```python
from build123d import *

# Parameters (mm, degrees)
SKETCH_W        = 230
SKETCH_H        = 140
PAD_DEPTH       = 40
SKETCH001_W     = 222
SKETCH001_H     = 132
POCKET_DEPTH    = 36
SKETCH002_W     = 98
SKETCH002_H     = 40
POCKET001_DEPTH = 5
SKETCH003_W     = 18
SKETCH003_H     = 12
POCKET002_DEPTH = 5
SKETCH004_W     = 15
SKETCH004_H     = 15
POCKET003_DEPTH = 5
SKETCH005_R     = 5
SKETCH005_R_2   = 1.9
PAD001_DEPTH    = 5
CHAMFER_SIZE    = 2


with BuildPart() as part:
    # Sketch → Pad (new body)
    with BuildSketch(Plane.XY):
        with Locations((115, 70)):
            Rectangle(SKETCH_W, SKETCH_H)
    extrude(amount=PAD_DEPTH)

    # Sketch001 (on Face6 of Pad) → Pocket (cut)
    with BuildSketch(Plane.XY.offset(40)):
        with Locations((115, 70)):
            Rectangle(SKETCH001_W, SKETCH001_H)
    extrude(amount=-POCKET_DEPTH, mode=Mode.SUBTRACT)

    # Sketch002 (on Face4 of Pocket) → Pocket001 (cut)
    with BuildSketch(Plane(origin=(0, 0, 0), x_dir=(1, 0, 0), z_dir=(0, 0, -1))):
        with Locations((171, -40)):
            Rectangle(SKETCH002_W, SKETCH002_H)
    extrude(amount=-POCKET001_DEPTH, mode=Mode.SUBTRACT)

    # Sketch003 (on Face2 of Pocket001) → Pocket002 (cut)
    with BuildSketch(Plane(origin=(0, 0, 0), x_dir=(0, -1, 0), z_dir=(-1, 0, 0))):
        with Locations((-114, 15)):
            Rectangle(SKETCH003_W, SKETCH003_H)
    extrude(amount=-POCKET002_DEPTH, mode=Mode.SUBTRACT)

    # Sketch004 (on Face6 of Pocket002) → Pocket003 (cut)
    with BuildSketch(Plane(origin=(0, 140, 0), x_dir=(-1, 0, 0), z_dir=(0, 1, 0))):
        with Locations((-197.5, 20)):
            Rectangle(SKETCH004_W, SKETCH004_H)
    extrude(amount=-POCKET003_DEPTH, mode=Mode.SUBTRACT)

    # Sketch005 (on Face23 of Pocket003) → Pad001 (join)
    with BuildSketch(Plane.XY.offset(4)):
        with Locations((217.5, 12.5)):
            Circle(SKETCH005_R)
        with Locations((217.5, 12.5)):
            Circle(SKETCH005_R_2, mode=Mode.SUBTRACT)
        with Locations((124.5, 12.5)):
            Circle(SKETCH005_R)
        with Locations((124.5, 12.5)):
            Circle(SKETCH005_R_2, mode=Mode.SUBTRACT)
        with Locations((217.5, 67.5)):
            Circle(SKETCH005_R)
        with Locations((217.5, 67.5)):
            Circle(SKETCH005_R_2, mode=Mode.SUBTRACT)
        with Locations((124.5, 67.5)):
            Circle(SKETCH005_R)
        with Locations((124.5, 67.5)):
            Circle(SKETCH005_R_2, mode=Mode.SUBTRACT)
        with Locations((15, 127.5)):
            Circle(SKETCH005_R)
        with Locations((15, 127.5)):
            Circle(SKETCH005_R_2, mode=Mode.SUBTRACT)
        with Locations((65, 127.5)):
            Circle(SKETCH005_R)
        with Locations((65, 127.5)):
            Circle(SKETCH005_R_2, mode=Mode.SUBTRACT)
        with Locations((65, 103.5)):
            Circle(SKETCH005_R)
        with Locations((65, 103.5)):
            Circle(SKETCH005_R_2, mode=Mode.SUBTRACT)
        with Locations((15, 103.5)):
            Circle(SKETCH005_R)
        with Locations((15, 103.5)):
            Circle(SKETCH005_R_2, mode=Mode.SUBTRACT)
        with Locations((15, 63)):
            Circle(SKETCH005_R)
        with Locations((15, 63)):
            Circle(SKETCH005_R_2, mode=Mode.SUBTRACT)
        with Locations((15, 15)):
            Circle(SKETCH005_R)
        with Locations((15, 15)):
            Circle(SKETCH005_R_2, mode=Mode.SUBTRACT)
        with Locations((83, 15)):
            Circle(SKETCH005_R)
        with Locations((83, 15)):
            Circle(SKETCH005_R_2, mode=Mode.SUBTRACT)
        with Locations((83, 63)):
            Circle(SKETCH005_R)
        with Locations((83, 63)):
            Circle(SKETCH005_R_2, mode=Mode.SUBTRACT)
        with Locations((85, 127.5)):
            Circle(SKETCH005_R)
        with Locations((85, 127.5)):
            Circle(SKETCH005_R_2, mode=Mode.SUBTRACT)
        with Locations((85, 101.5)):
            Circle(SKETCH005_R)
        with Locations((85, 101.5)):
            Circle(SKETCH005_R_2, mode=Mode.SUBTRACT)
        with Locations((151, 101.5)):
            Circle(SKETCH005_R)
        with Locations((151, 101.5)):
            Circle(SKETCH005_R_2, mode=Mode.SUBTRACT)
        with Locations((151, 127.5)):
            Circle(SKETCH005_R)
        with Locations((151, 127.5)):
            Circle(SKETCH005_R_2, mode=Mode.SUBTRACT)
    extrude(amount=PAD001_DEPTH)

    # Chamfer
    chamfer_edges = [part.edges().sort_by_distance(p)[0] for p in [
        (0, 140, 20),
        (115, 140, 0),
        (230, 140, 20),
        (230, 70, 0),
        (230, 0, 20),
        (115, 0, 0),
        (0, 0, 20),
        (0, 70, 0),
    ]]
    chamfer(chamfer_edges, length=CHAMFER_SIZE)


solid = part.part
```
Geometry check sheet. Reference: the model listing, model coordinates, mm. Round coordinates to 2 decimals unless told otherwise and drop trailing zeros. Loops run counter-clockwise (first coordinate to the right, second up) from the corner with the lowest first, then second, coordinate; pieces in that order, holes last. Notation, with made-up numbers: (23.5, 62.5) - (53.5, 62.5) arc R6 ccw to (53.5, 72.5) - close; hole circle Ø5 at (38.25, -10.75). An arc over 180 degrees is marked (long way). Write each question's results on one line, items separated by ' | '. Start each with the question number.
Q1. Cross-section at C-C on x = 23.5. Enter the section's corners in (y, z), and give its area (3 significant figures).
Q2. Cross-section at A-A on z = 15. Enter the section's corners in (x, y), and give its area (3 significant figures).
Q3. Thickness scan on line 1 (Y direction, x = 151, z = 6); line 2 (Y direction, x = 124.5, z = 5.75); line 3 (X direction, y = 19, z = 17). Record the ranges inside material, lowest first. Write a range as [from, to].
Q4. Gauge pin test, flat ends, axial feed: P1, Ø1.5, axis at x = 155.5, y = 59.5, coming from the +Z side; P2, Ø3, axis at x = 219, y = 67, coming from the +Z side; P3, Ø12, axis at x = 184, y = 27, coming from the +Z side. Record the tip position at first contact, or that the pin passes through.
Q5. Release check for a two-part mould opening along X. For faces 1 (the flat face through (113, 0, 21)), 2 (the cylindrical face through (87.619, 13.085, 6.465)) record: +X half, -X half, draft (parallel to the pull), parting line (faces both ways), or undercut.
Q6. Cross-section at B-B on y = 36. Enter the section's corners in (x, z), and give its area (3 significant figures).
Answers below:
1) outline: (0, 2) - (2, 0) - (138, 0) - (140, 2) - (140, 40) - (136, 40) - (136, 4) - (4, 4) - (4, 40) - (0, 40) - close | area: 844 mm²
2) outline: (0, 2) - (2, 0) - (228, 0) - (230, 2) - (230, 138) - (228, 140) - (205, 140) - (205, 136) - (226, 136) - (226, 4) - (4, 4) - (4, 105) - (0, 105) - close; (0, 123) - (4, 123) - (4, 136) - (190, 136) - (190, 140) - (2, 140) - (0, 138) - close | area: 2,760 mm²
3) line 1: y = [0, 4], [96.5, 99.6], [103.4, 106.5], [122.5, 125.6], [129.4, 132.5], [136, 140] | line 2: y = [0, 4], [7.5, 10.6], [14.4, 17.5], [62.5, 65.6], [69.4, 72.5], [136, 140] | line 3: x = [0, 4], [226, 230]
4) P1: stops at z = 4 | P2: stops at z = 9 | P3: passes through
5) face 1: draft | face 2: undercut
6) outline: (0, 2) - (2, 0) - (122, 0) - (122, 4) - (4, 4) - (4, 40) - (0, 40) - close; (220, 0) - (228, 0) - (230, 2) - (230, 40) - (226, 40) - (226, 4) - (220, 4) - close | area: 812 mm²
